Job drawing, mm, ordinate dimensions from the low corner. One solid piece. Give positions to 0.01 mm unless a question says otherwise; leave off trailing zeros. Loops run counter-clockwise (first coordinate to the right, second up) from the corner with the lowest first, then second, coordinate; pieces in that order, holes last.
Item 1: Probe probe 1 along Y at (x, z) = (2.7, 33) (1 decimal); probe 2 along Y at (x, z) = (1.3, 31) (1 decimal); probe 3 along Z at (x, y) = (1.1, 30.48) (1 decimal). List the from-to ranges inside material, lowest first.
Item 2: Saw through at C-C on x = 2.2. Give the number of separate pieces and of enclosed holes in the cut face, plus the area to 3 significant figures.
Item 3: Saw through at D-D on y = 48.5. Give the cut face in (x, z).
Item 4: Saw through at A-A on y = 30.48. Give the cut face in (x, z) (1 decimal).
Item 5: Drop flat-ended pins along their axis: P1, Ø9.5, axis at y = 55.81, z = 26.71, coming from the -X side; P2, Ø5, axis at y = 5.15, z = 30.51, coming from the +X side; P3, Ø1, axis at x = 2.5, z = 27.5, coming from the +Y side. Give the stop position or say it passes through.
Item 6: Saw through at B-B on z = 4. Give the cut face in (x, y).
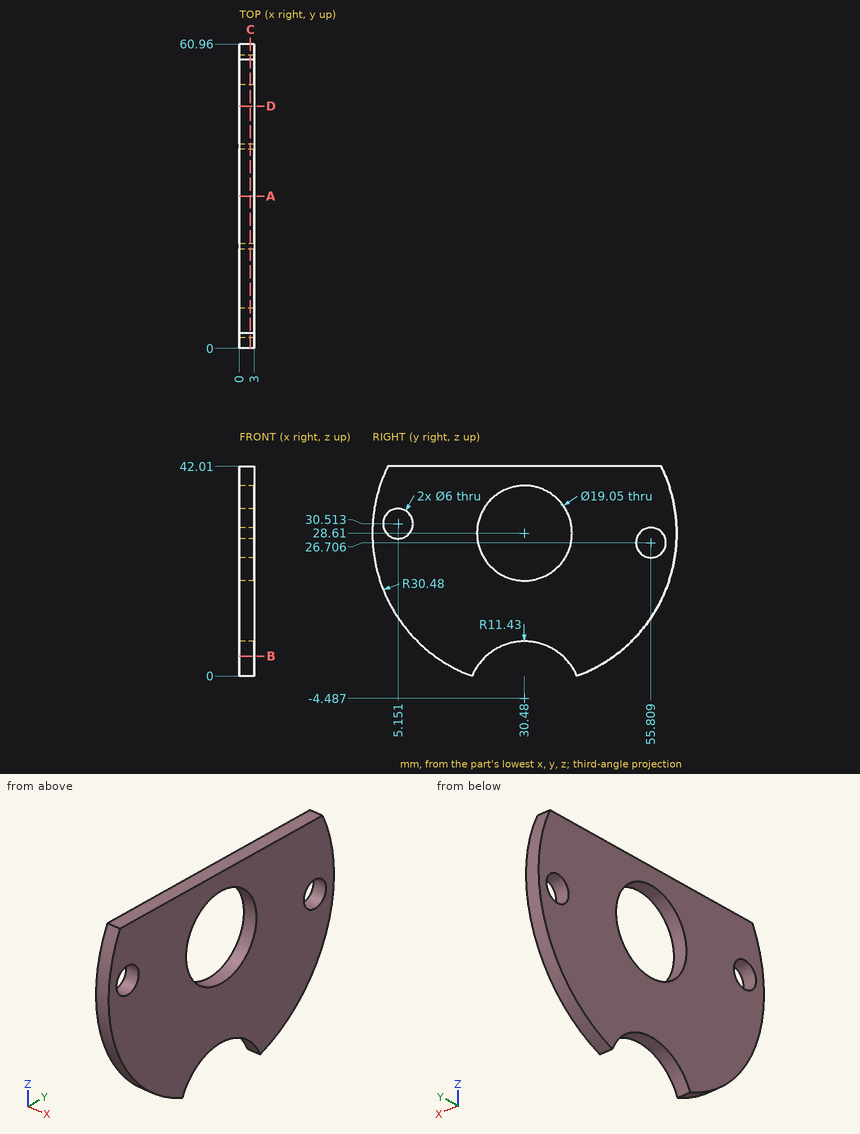
Results below:
1. probe 1: y = 0.3 to 3.5, 6.8 to 22, 38.9 to 60.6
1. probe 2: y = 0.1 to 2.2, 8.1 to 21.3, 39.7 to 60.9
1. probe 3: z = 6.9 to 19.1, 38.1 to 42
2. separate pieces: 1
2. enclosed holes: 3
2. area: 1,780 mm2
3. outline: (0, 4.03) - (3, 4.03) - (3, 42.01) - (0, 42.01) - close
4. outline: (0, 6.9) - (3, 6.9) - (3, 19.1) - (0, 19.1) - close; (0, 38.1) - (3, 38.1) - (3, 42) - (0, 42) - close
5. P1: stops at x = 0
5. P2: passes through
5. P3: stops at y = 60.95
6. outline: (0, 12.5) - (3, 12.5) - (3, 22.82) - (0, 22.82) - close; (0, 38.14) - (3, 38.14) - (3, 48.46) - (0, 48.46) - close
